Input: part model. Units: mm. Frame: model coordinates. A direction names the side the tool comes from. Coordinates: 2 decimals unless noted, no trailing zeros. Order: outer loops, then holes, each group sorted by start corner. A loop starts at its lowest first (then second) coordinate and runs counter-clockwise, first axis right, second up. Notation, with made-up numbers: (54, 73) - (79, 73) arc R24 ccw to (79, 102) - close; hole circle Ø11 at (-30, 18). An arc over 180 degrees is marked (long way). Answer as CSV lines item,"result". Start each with the question number.
Item 1: Draft query along Y for faces 6 (the flat face through (50, 0, 2)), 7 (the flat face through (3.2, 47, 2)), 8 (the flat face through (64, 41, 0)). Return one class per face: +Y half, -Y half, draft (parallel to the pull), parting line (faces both ways), or undercut.
Item 2: Access query for faces 1 (the flat face through (128, 66.767, 2)), 2 (the flat face through (2, 13.233, 2)), 3 (the flat face through (130, 47, 2)), 4 (the flat face through (128, 13.433, 2)), 5 (the flat face through (36, 3.2, 2)). Directions: +Z, -Z, +X, -X, +Y, -Y. A direction counts if a zero-diameter tool reaches every point of the face in a straight line with its end or side. Return the directions, or none.
Item 3: Section A-A (y = 74.5). Output: boundary loops of the cut face in (x, z), and give its area (3 significant figures).
Item 4: Section C-C (x = 91.5). Output: boundary loops of the cut face in (y, z), and give its area (3 significant figures).
Item 5: First-contact query: pin 1 (1.6 mm diameter, centred on x = 1, z = 1.5, fed in from -Y); pin 2 (1.6 mm diameter, centred on y = 71, z = 1, fed in from -X); pin 3 (1.6 mm diameter, centred on x = 2, z = 2.5, fed in from +Y). Flat tips, straight axial feed; report the tip coordinate or a pass-through.
Item 6: Material intervals for line 1 along X through (y, z) = (74.5, 1.75); line 2 along Y through (x, z) = (15.2, 0.75); line 3 along X through (y, z) = (50.5, 2.5), sorted ascending.
Item 7: Section B-B (z = 2.3). State how many separate pieces and enclosed holes the cut face has, and give its area (3 significant figures).
from build123d import *

# Parameters (mm, degrees)
SKETCH1_W           = 130
SKETCH1_H           = 80
BOSS_EXTRUDE1_DEPTH = 3.2
SKETCH2_W           = 14.444444444
SKETCH2_H           = 3.2
SKETCH2_W_2         = 3.2
SKETCH2_H_2         = 13.333333334
SKETCH2_H_3         = 13.333333333
CUT_EXTRUDE1_DEPTH  = 153.676913775
MOVE_FACE1_BY       = 0.1
MOVE_FACE1_2_BY     = 0.1
MOVE_FACE1_3_BY     = 0.1
MOVE_FACE1_4_BY     = 0.1
MOVE_FACE1_5_BY     = 0.1
MOVE_FACE1_6_BY     = 0.1
MOVE_FACE1_7_BY     = 0.1
MOVE_FACE1_8_BY     = 0.1
MOVE_FACE1_9_BY     = 0.1
MOVE_FACE1_10_BY    = 0.1
MOVE_FACE1_11_BY    = 0.1
MOVE_FACE1_12_BY    = 0.1
MOVE_FACE1_13_BY    = 0.1
MOVE_FACE1_14_BY    = 0.1
MOVE_FACE1_15_BY    = 0.1
MOVE_FACE1_16_BY    = 0.1
MOVE_FACE1_17_BY    = 0.1
MOVE_FACE1_18_BY    = 0.1
CUT_EXTRUDE2_REACH  = 154.677
SKETCH3_R           = 1.7
CUT_EXTRUDE3_REACH  = 154.677


with BuildPart() as part:
    # Sketch1 → Boss-Extrude1 (new body)
    with BuildSketch(Plane.XY):
        with Locations((65, 40)):
            Rectangle(SKETCH1_W, SKETCH1_H)
    extrude(amount=BOSS_EXTRUDE1_DEPTH)

    # Sketch2 → Cut-Extrude1 (cut, through all)
    with BuildSketch(Plane.XY.offset(3.2)):
        with Locations((7.222222222, 1.6)):
            Rectangle(SKETCH2_W, SKETCH2_H)
        with Locations((36.111111111, 1.6)):
            Rectangle(SKETCH2_W, SKETCH2_H)
        with Locations((65, 1.6)):
            Rectangle(SKETCH2_W, SKETCH2_H)
        with Locations((93.888888889, 1.6)):
            Rectangle(SKETCH2_W, SKETCH2_H)
        Polygon((115.555555556, 0), (115.555555556, 3.2), (126.8, 3.2), (126.8, 13.333333333), (130, 13.333333333), (130, 0), align=None)
        with Locations((1.6, 20)):
            Rectangle(SKETCH2_W_2, SKETCH2_H_2)
        with Locations((1.6, 46.666666667)):
            Rectangle(SKETCH2_W_2, SKETCH2_H_3)
        with Locations((1.6, 73.333333334)):
            Rectangle(SKETCH2_W_2, SKETCH2_H_3)
        with Locations((128.4, 33.333333334)):
            Rectangle(SKETCH2_W_2, SKETCH2_H_3)
        with Locations((128.4, 60)):
            Rectangle(SKETCH2_W_2, SKETCH2_H_2)
    extrude(amount=-CUT_EXTRUDE1_DEPTH, mode=Mode.SUBTRACT)

    # Move Face1: a face moved inward by 0.1
    extrude(part.faces().sort_by_distance((128.4, 53.333333333, 1.6))[0], amount=MOVE_FACE1_BY, dir=(0, -1, 0), mode=Mode.SUBTRACT)

    # Move Face1 2: a face moved inward by 0.1
    extrude(part.faces().sort_by_distance((128.4, 26.666666667, 1.6))[0], amount=MOVE_FACE1_2_BY, dir=(0, -1, 0), mode=Mode.SUBTRACT)

    # Move Face1 3: a face moved inward by 0.1
    extrude(part.faces().sort_by_distance((128.4, 13.333333333, 1.6))[0], amount=MOVE_FACE1_3_BY, dir=(0, 1, 0), mode=Mode.SUBTRACT)

    # Move Face1 4: a face moved inward by 0.1
    extrude(part.faces().sort_by_distance((128.4, 40, 1.6))[0], amount=MOVE_FACE1_4_BY, dir=(0, 1, 0), mode=Mode.SUBTRACT)

    # Move Face1 5: a face moved inward by 0.1
    extrude(part.faces().sort_by_distance((128.4, 66.666666667, 1.6))[0], amount=MOVE_FACE1_5_BY, dir=(0, 1, 0), mode=Mode.SUBTRACT)

    # Move Face1 6: a face moved inward by 0.1
    extrude(part.faces().sort_by_distance((115.555555556, 1.6, 1.6))[0], amount=MOVE_FACE1_6_BY, dir=(-1, 0, 0), mode=Mode.SUBTRACT)

    # Move Face1 7: a face moved inward by 0.1
    extrude(part.faces().sort_by_distance((86.666666667, 1.6, 1.6))[0], amount=MOVE_FACE1_7_BY, dir=(-1, 0, 0), mode=Mode.SUBTRACT)

    # Move Face1 8: a face moved inward by 0.1
    extrude(part.faces().sort_by_distance((57.777777778, 1.6, 1.6))[0], amount=MOVE_FACE1_8_BY, dir=(-1, 0, 0), mode=Mode.SUBTRACT)

    # Move Face1 9: a face moved inward by 0.1
    extrude(part.faces().sort_by_distance((28.888888889, 1.6, 1.6))[0], amount=MOVE_FACE1_9_BY, dir=(-1, 0, 0), mode=Mode.SUBTRACT)

    # Move Face1 10: a face moved inward by 0.1
    extrude(part.faces().sort_by_distance((14.444444444, 1.6, 1.6))[0], amount=MOVE_FACE1_10_BY, dir=(1, 0, 0), mode=Mode.SUBTRACT)

    # Move Face1 11: a face moved inward by 0.1
    extrude(part.faces().sort_by_distance((43.333333333, 1.6, 1.6))[0], amount=MOVE_FACE1_11_BY, dir=(1, 0, 0), mode=Mode.SUBTRACT)

    # Move Face1 12: a face moved inward by 0.1
    extrude(part.faces().sort_by_distance((72.222222222, 1.6, 1.6))[0], amount=MOVE_FACE1_12_BY, dir=(1, 0, 0), mode=Mode.SUBTRACT)

    # Move Face1 13: a face moved inward by 0.1
    extrude(part.faces().sort_by_distance((101.111111111, 1.6, 1.6))[0], amount=MOVE_FACE1_13_BY, dir=(1, 0, 0), mode=Mode.SUBTRACT)

    # Move Face1 14: a face moved inward by 0.1
    extrude(part.faces().sort_by_distance((1.6, 26.666666667, 1.6))[0], amount=MOVE_FACE1_14_BY, dir=(0, 1, 0), mode=Mode.SUBTRACT)

    # Move Face1 15: a face moved inward by 0.1
    extrude(part.faces().sort_by_distance((1.6, 13.333333333, 1.6))[0], amount=MOVE_FACE1_15_BY, dir=(0, -1, 0), mode=Mode.SUBTRACT)

    # Move Face1 16: a face moved inward by 0.1
    extrude(part.faces().sort_by_distance((1.6, 40, 1.6))[0], amount=MOVE_FACE1_16_BY, dir=(0, -1, 0), mode=Mode.SUBTRACT)

    # Move Face1 17: a face moved inward by 0.1
    extrude(part.faces().sort_by_distance((1.6, 53.333333333, 1.6))[0], amount=MOVE_FACE1_17_BY, dir=(0, 1, 0), mode=Mode.SUBTRACT)

    # Move Face1 18: a face moved inward by 0.1
    extrude(part.faces().sort_by_distance((1.6, 66.666666667, 1.6))[0], amount=MOVE_FACE1_18_BY, dir=(0, -1, 0), mode=Mode.SUBTRACT)

    # Sketch3 → Cut-Extrude2 (cut, up to next)
    with BuildSketch(Plane.XY.offset(3.2), mode=Mode.PRIVATE) as cut_extrude2_sk1:
        with Locations((15.2, 74.5)):
            Circle(SKETCH3_R)
    cut_extrude2_tool1 = extrude(cut_extrude2_sk1.sketch, amount=-CUT_EXTRUDE2_REACH, mode=Mode.PRIVATE) & part.part
    # Sketch3 → Cut-Extrude2 (cut, up to next)
    with BuildSketch(Plane.XY.offset(3.2), mode=Mode.PRIVATE) as cut_extrude2_sk2:
        with Locations(Location((114.8, 74.5, 0), (0, 0, 180))):
            Circle(SKETCH3_R)
    cut_extrude2_tool2 = extrude(cut_extrude2_sk2.sketch, amount=-CUT_EXTRUDE2_REACH, mode=Mode.PRIVATE) & part.part
    add(cut_extrude2_tool1.solids().sort_by_distance((15.2, 74.5, 3.2))[0], mode=Mode.SUBTRACT)
    add(cut_extrude2_tool2.solids().sort_by_distance((114.8, 74.5, 3.2))[0], mode=Mode.SUBTRACT)

    # Sketch4 → Cut-Extrude3 (cut, up to next)
    with BuildSketch(Plane(origin=(0, 0, 0), x_dir=(-1, 0, 0), z_dir=(0, 0, -1)), mode=Mode.PRIVATE) as cut_extrude3_sk1:
        with BuildLine():
            Line((-97.788888889, 3.2), (-97.788888889, 7.1))
            ThreePointArc((-97.788888889, 7.1), (-93.888888889, 11), (-89.988888889, 7.1))
            Line((-89.988888889, 7.1), (-89.988888889, 3.2))
            Line((-89.988888889, 3.2), (-97.788888889, 3.2))
        make_face()
    cut_extrude3_tool1 = extrude(cut_extrude3_sk1.sketch, amount=-CUT_EXTRUDE3_REACH, mode=Mode.PRIVATE) & part.part
    add(cut_extrude3_tool1.solids().sort_by_distance((93.888889, 6.735936, 0))[0], mode=Mode.SUBTRACT)


solid = part.part
Determined:
1,face 6,"-Y half"
1,face 7,"undercut"
1,face 8,"draft"
2,face 1,"+Z, -Z, +X"
2,face 2,"+Z, -Z, -X"
2,face 3,"+Z, -Z, +X, +Y, -Y"
2,face 4,"+Z, -Z, +X, -Y"
2,face 5,"+Z, -Z, -Y"
3,outline,"(3.2, 0) - (13.5, 0) - (13.5, 3.2) - (3.2, 3.2) - close; (16.9, 0) - (113.1, 0) - (113.1, 3.2) - (16.9, 3.2) - close; (116.5, 0) - (130, 0) - (130, 3.2) - (116.5, 3.2) - close"
3,area,"384 mm^2"
4,outline,"(10.18, 0) - (80, 0) - (80, 3.2) - (10.18, 3.2) - close"
4,area,"223 mm^2"
5,pin 1,"stops at y = 3.2"
5,pin 2,"stops at x = 3.2"
5,pin 3,"stops at y = 66.57"
6,line 1,"x = 3.2 to 13.5, 16.9 to 113.1, 116.5 to 130"
6,line 2,"y = 0 to 72.8, 76.2 to 80"
6,line 3,"x = 3.2 to 130"
7,separate pieces,"1"
7,enclosed holes,"2"
7,area,"9,840 mm^2"
